Autodesk Inventor part; units mm, degrees
ref_plane "YZ Plane" through (0, 0, 0) normal (1, 0, 0) x (0, 1, 0)
ref_plane "XZ Plane" through (0, 0, 0) normal (0, 1, 0) x (-1, 0, 0)
ref_plane "XY Plane" through (0, 0, 0) normal (0, 0, 1) x (1, 0, 0)
sketch "Sketch7" plane through (0, 0, 0) normal (0, 0, 1) x (1, 0, 0)
  line L0 (240, 10) -> (-240, 10)
  line L1 (-240, 10) -> (-240, -10)
  line L2 (-240, -10) -> (240, -10)
  line L3 (240, -10) -> (240, 10)
  line L4 (240, 10) -> (-240, -10) construction
  line L5 (-240, 10) -> (240, -10) construction
  point P0 (0, 0)
  dimension "d52" = 480
  dimension "d53" = 20
extrude "Plate6" add sketch "Sketch7" along normal blind 2
sketch "Sketch8" plane through (-240, -8.0167, 1.7423) normal (0, -0.9916667, 0.1288302) x (1, 0, 0)
  line L0 (480, 0) -> (0, 0)
  line L1 (0, 0) -> (0, -100)
  line L2 (0, -100) -> (480, -100)
  line L3 (480, -100) -> (480, 0)
edge flange "Flange5" height 100 angle 82.598 thickness 2 bend radius 2.75 thickness toward (0, -0.9916667, 0.1288302) relief round relief width 2 relief depth 1 edges at (0, -10, 0) wall of the first edge with corners at (240, -8.0167, 1.7423) (-240, -8.0167, 1.7423) (-240, -20.8997, -97.4243) (240, -20.8997, -97.4243)
bend "Bend5"
corner "Corner5"
equation "\"d54\" = Thickness"
equation "\"d55\" = BendReliefWidth"
equation "\"d56\" = BendReliefDepth"
equation "\"d57\" = MinimumRemnant"
equation "\"d58\" = TransitionRadius"
equation "\"d61\" = BendRadius"
equation "\"d62\" = CornerReliefSize"
equation "\"d63\" = GapSize"
equation "\"d64\" = JacobiRadiusSize"
equation "\"BendReliefWidth\" = Thickness"
equation "\"BendReliefDepth\" = 0.5 * Thickness"
equation "\"CornerReliefSize\" = 4 * Thickness"
equation "\"MinimumRemnant\" = 2 * Thickness"
equation "\"TransitionRadius\" = BendRadius"
equation "\"JacobiRadiusSize\" = BendRadius"
equation "\"GapSize\" = Thickness"
properties part number "TRM 017 sheet in" material "AISI 304"
The model under review builds one solid part; all positions refer to its coordinate system, in mm. A direction names the side the tool comes from. Coordinates: 2 decimals unless noted, no trailing zeros. Order: outer loops, then holes, each group sorted by start corner. A loop starts at its lowest first (then second) coordinate and runs counter-clockwise, first axis right, second up. Notation, with made-up numbers: (68, -17) -> (98, -17) arc R24 cw to (98, 7) -> close; hole circle Ø4 at (17, 62.25). An arc over 180 degrees is marked (long way). Answer in a Markdown table with one row per item. Add a question column.
Item 1: Machinability: for faces 1 (the flat face through (-3, 2, 0)), 2 (the flat face through (-3, 2, 2)), which of the approach directions +Z, -Z, +X, -X, +Y, -Y give a long, thin tool a straight path to every point of the face, cutting with its end or side? Answer none if there is none.
Item 2: Clearance check with flat-ended pins moving along their axes: pin 1 (10 mm diameter, centred on x = -2, z = -29, fed in from -Y); pin 2 (6 mm diameter, centred on x = 14, z = -70, fed in from -Y); pin 3 (17.5 mm diameter, centred on x = 8.5, y = 5, fed in from -Z). State where each tip first meets the part, or that it passes through.
Item 3: We need section C-C on z = -64.5. Write out the cut boundary in (x, y), plus the area to 3 significant figures.
Item 4: To check wall thickness, follow probe 1 along Z at (x, y) = (65.5, -0.5); probe 2 along Z at (x, y) = (142.5, -8); probe 3 along Y at (x, z) = (64, -44). State the ranges of each line that lie inside material, in increasing order.
Item 5: We need section A-A on x = 191. Write out the cut boundary in (y, z), plus the area to 3 significant figures.
Item 6: We need section B-B on y = 0. Write out the cut boundary in (x, z).
Final values:
| question | item | result |
|---|---|---|
| 1 | face 1 | -Z, +X, -X, +Y |
| 1 | face 2 | +Z, +X, -X, +Y, -Y |
| 2 | pin 1 | stops at y = -14.68 |
| 2 | pin 2 | stops at y = -19.74 |
| 2 | pin 3 | stops at z = 0 |
| 3 | outline | (-240, -18.64) -> (240, -18.64) -> (240, -16.62) -> (-240, -16.62) -> close |
| 3 | area | 968 mm2 |
| 4 | probe 1 | z = 0 to 2 |
| 4 | probe 2 | z = -1.06 to 1.47 |
| 4 | probe 3 | y = -15.98 to -13.96 |
| 5 | outline | (-22.88, -97.17) -> (-20.9, -97.42) -> (-8.55, -2.4) arc R2.75 cw to (-5.83, 0) -> (10, 0) -> (10, 2) -> (-5.83, 2) arc R4.75 ccw to (-10.54, -2.14) -> close |
| 5 | area | 234 mm2 |
| 6 | outline | (-240, 0) -> (240, 0) -> (240, 2) -> (-240, 2) -> close |
